Verification items for the finished model (mm, model axes). Coordinates: 2 decimals unless noted, no trailing zeros. Write each loop counter-clockwise with the first axis right and the second up, starting at its lowest first coordinate (ties: lowest second). Pieces come first, ordered by that corner, then holes. Notation, with made-up numbers: (64, 33.25) -> (70, 33.25) arc R30 cw to (70, 68.25) -> close; hole circle Ø6 at (6, 36.25). An arc over 180 degrees is marked (long way). Answer in a Markdown table with one row per item.
```python
from build123d import *

# Parameters (mm, degrees)
CYLINDER038_R       = 1.8
CYLINDER038_DEPTH   = 10
ARRAY001019_X_COUNT = 2
ARRAY001019_X_PITCH = 20
ARRAY001019_Z_COUNT = 2
ARRAY001019_Z_PITCH = 114
BOX018_W            = 30
BOX018_H            = 3
BOX018_DEPTH        = 124


with BuildPart() as side_connector_hole_array:
    # Cylinder038 → Cylinder038 (new body)
    with BuildSketch(Plane.XZ):
        Circle(CYLINDER038_R)
    extrude(amount=CYLINDER038_DEPTH)

    # Array001019 X: side connector hole array ×2


with BuildPart() as side_connector_hole_array_1:
    add(side_connector_hole_array.part)
    with Locations(*[(i * ARRAY001019_X_PITCH, 0, 0) for i in range(1, ARRAY001019_X_COUNT)]):
        add(side_connector_hole_array.part)

    # Array001019 Z: side connector hole array ×2


with BuildPart() as side_connector_hole_array_2:
    add(side_connector_hole_array_1.part)
    with Locations(*[(0, 0, i * ARRAY001019_Z_PITCH) for i in range(1, ARRAY001019_Z_COUNT)]):
        add(side_connector_hole_array_1.part)


with BuildPart() as side_connector_hole_array_3:
    # Array001019 placement: moved
    add(side_connector_hole_array_2.part.moved(Location((5, 5, 5))))


with BuildPart() as vertical_side_connector_clone002:
    # Box018 → Box018 (new body)
    with BuildSketch(Plane.XY):
        with Locations((15, 1.5)):
            Rectangle(BOX018_W, BOX018_H)
    extrude(amount=BOX018_DEPTH)

    # Cut014: cut side connector hole array
    add(side_connector_hole_array_3.part, mode=Mode.SUBTRACT)


with BuildPart() as vertical_side_connector_clone002_1:
    # Compound001 placement: moved
    add(vertical_side_connector_clone002.part.moved(Location((0, -11, -36))))


with BuildPart() as vertical_side_connector_clone002_2:
    # Clone006 placement: moved
    add(vertical_side_connector_clone002_1.part.moved(Location((0, 6, 2))))


with BuildPart() as vertical_side_connector_clone002_3:
    # Body006 placement: moved
    add(vertical_side_connector_clone002_2.part.moved(Location((114, 95, -2))))


solid = vertical_side_connector_clone002_3.part
```
1. Section check A-A, the plane x = 119. Record the boundary of the cut face in (y, z).
Geometry says:
| item | result |
|---|---|
| outline | (90, -36) -> (93, -36) -> (93, -32.8) -> (90, -32.8) -> close; (90, -29.2) -> (93, -29.2) -> (93, 81.2) -> (90, 81.2) -> close; (90, 84.8) -> (93, 84.8) -> (93, 88) -> (90, 88) -> close |
2. Mould release check, pull along X, two halves, no side actions. Record for faces 1 (the flat face through (129, 92, 88)), 2 (the cylindrical face through (117.2, 91.52, 83.08)), 3 (the flat face through (114, 91, 25)): released by +X, released by -X, zero draft, split by the parting line, or undercut.
Geometry says:
| item | result |
|---|---|
| face 1 | zero draft |
| face 2 | undercut |
| face 3 | released by -X |
3. Section check B-B, the plane z = 83. Record the boundary of the cut face in (x, y).
Geometry says:
| item | result |
|---|---|
| outline | (114, 90) -> (117.2, 90) -> (117.2, 93) -> (114, 93) -> close; (120.8, 90) -> (137.2, 90) -> (137.2, 93) -> (120.8, 93) -> close; (140.8, 90) -> (144, 90) -> (144, 93) -> (140.8, 93) -> close |
4. Depth check by flat-ended pin: P1, Ø4, axis at x = 139, z = -31, coming from the -Y side. Enter the tip coordinate at first touch or a pass-through.
Geometry says:
| item | result |
|---|---|
| P1 | y = 90 |
5. Thickness scan on line 1 (Z direction, x = 139, y = 90.8); line 2 (X direction, y = 92.05, z = -31); line 3 (Z direction, x = 139.75, y = 90.7). Record the ranges inside material, lowest first. Write a range as from..to.
Geometry says:
| item | result |
|---|---|
| line 1 | -36..-32.8, -29.2..81.2, 84.8..88 |
| line 2 | 114..117.2, 120.8..137.2, 140.8..144 |
| line 3 | -36..-32.64, -29.36..81.36, 84.64..88 |
